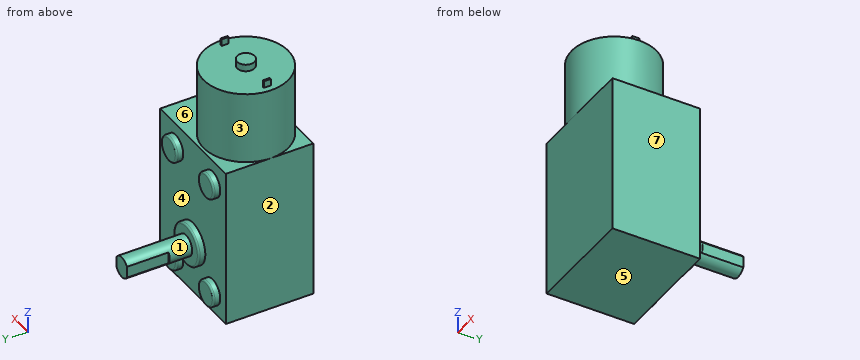
from build123d import *

# Parameters (mm, degrees)
CROQUIS1_W              = 32
CROQUIS1_H              = 46
CROQUIS1_R              = 6
CROQUIS1_R_2            = 3.7
SALIENTE_EXTRUIR1_DEPTH = 25.2
CROQUIS2_R              = 3.7
CROQUIS2_R_2            = 6
SALIENTE_EXTRUIR2_DEPTH = 2
CROQUIS3_R              = 12.2
SALIENTE_EXTRUIR3_DEPTH = 20.8
CROQUIS4_R              = 2.5
SALIENTE_EXTRUIR4_DEPTH = 2
CROQUIS5_W              = 0.5
CROQUIS5_H              = 2
SALIENTE_EXTRUIR5_DEPTH = 2
CROQUIS6_R              = 3
SALIENTE_EXTRUIR6_DEPTH = 18.5
CORTAR_EXTRUIR1_DEPTH   = 12
REDONDEO2_R             = 0.5


with BuildPart() as part:
    # Croquis1 → Saliente-Extruir1 (new body)
    with BuildSketch(Plane(origin=(0, 0, 0), x_dir=(1, 0, 0), z_dir=(0, 1, 0))):
        Rectangle(CROQUIS1_W, CROQUIS1_H)
        with Locations((0, 8)):
            Circle(CROQUIS1_R, mode=Mode.SUBTRACT)
        with Locations((8.430868167, -16)):
            Circle(CROQUIS1_R_2, mode=Mode.SUBTRACT)
        with Locations((-9.569131833, -16)):
            Circle(CROQUIS1_R_2, mode=Mode.SUBTRACT)
        with Locations((8.430868167, 17)):
            Circle(CROQUIS1_R_2, mode=Mode.SUBTRACT)
        with Locations((-9.569131833, 17)):
            Circle(CROQUIS1_R_2, mode=Mode.SUBTRACT)
        with Locations((0, 8)):
            Circle(CROQUIS1_R)
        with Locations((-9.569131833, 17)):
            Circle(CROQUIS1_R_2)
        with Locations((8.430868167, 17)):
            Circle(CROQUIS1_R_2)
        with Locations((-9.569131833, -16)):
            Circle(CROQUIS1_R_2)
        with Locations((8.430868167, -16)):
            Circle(CROQUIS1_R_2)
    extrude(amount=SALIENTE_EXTRUIR1_DEPTH)

    # Croquis2 → Saliente-Extruir2 (add)
    with BuildSketch(Plane(origin=(0, 25.2, 0), x_dir=(1, 0, 0), z_dir=(0, 1, 0))):
        with Locations((-9.569131833, 17)):
            Circle(CROQUIS2_R)
        with Locations((8.430868167, 17)):
            Circle(CROQUIS2_R)
        with Locations((8.430868167, -16)):
            Circle(CROQUIS2_R)
        with Locations((-9.569131833, -16)):
            Circle(CROQUIS2_R)
        with Locations((0, 8)):
            Circle(CROQUIS2_R_2)
    extrude(amount=SALIENTE_EXTRUIR2_DEPTH)

    # Croquis3 → Saliente-Extruir3 (add)
    with BuildSketch(Plane.XY.offset(23)):
        with Locations((-3.8, 12.2)):
            Circle(CROQUIS3_R)
    extrude(amount=SALIENTE_EXTRUIR3_DEPTH)

    # Croquis4 → Saliente-Extruir4 (add)
    with BuildSketch(Plane.XY.offset(43.8)):
        with Locations((-3.8, 12.2)):
            Circle(CROQUIS4_R)
    extrude(amount=SALIENTE_EXTRUIR4_DEPTH)

    # Croquis5 → Saliente-Extruir5 (add)
    with BuildSketch(Plane.XY.offset(43.8)):
        with Locations((6.559315441, 12.2)):
            Rectangle(CROQUIS5_W, CROQUIS5_H)
        with Locations((-13.968008184, 12.2)):
            Rectangle(CROQUIS5_W, CROQUIS5_H)
    extrude(amount=SALIENTE_EXTRUIR5_DEPTH)

    # Croquis6 → Saliente-Extruir6 (add)
    with BuildSketch(Plane(origin=(0, 27.2, 0), x_dir=(1, 0, 0), z_dir=(0, 1, 0))):
        with Locations((0, 8)):
            Circle(CROQUIS6_R)
    extrude(amount=SALIENTE_EXTRUIR6_DEPTH)

    # Croquis7 → Cortar-Extruir1 (cut)
    with BuildSketch(Plane(origin=(0, 45.7, 0), x_dir=(1, 0, 0), z_dir=(0, 1, 0))):
        with BuildLine():
            Line((-2.5, 6.341687605), (-2.5, 9.658312395))
            ThreePointArc((-2.5, 9.658312395), (-3, 8), (-2.5, 6.341687605))
        make_face()
        with BuildLine():
            Line((2.5, 6.341687605), (2.5, 9.658312395))
            ThreePointArc((2.5, 9.658312395), (3, 8), (2.5, 6.341687605))
        make_face()
    extrude(amount=-CORTAR_EXTRUIR1_DEPTH, mode=Mode.SUBTRACT)

    # Redondeo2
    redondeo2_edges = [part.edges().sort_by_distance(p)[0] for p in [
        (-13.269131833, 27.2, -17),
        (4.730868167, 27.2, -17),
        (4.730868167, 27.2, 16),
        (-13.269131833, 27.2, 16),
        (-6, 27.2, -8),
    ]]
    fillet(redondeo2_edges, radius=REDONDEO2_R)


solid = part.part
CAD build for the part. Positions are in the model's coordinates, mm. Face numbers are marked on the shaded views. A direction names the side the tool comes from. Give positions to 0.01 mm unless a question says otherwise; leave off trailing zeros. Write each loop counter-clockwise with the first axis right and the second up, starting at its lowest first coordinate (ties: lowest second). Pieces come first, ordered by that corner, then holes. Notation, with made-up numbers: (-38.75, 43) - (-17.75, 43) arc R16 ccw to (-17.75, 52) - close; hole circle Ø4 at (42, 4). An arc over 180 degrees is marked (long way). Put each result on its own line as item: value.
(1) Drop flat-ended pins along their axis: pin 1 Ø10 at (x, y) = (-7, 21.5) entering from +Z; pin 2 Ø7 at (x, z) = (-10.5, -16.5) entering from +Y; pin 3 Ø1.6 at (y, z) = (12.5, 45) entering from +X. Give the stop position or say it passes through.
Working result:
pin 1: z = 43.8
pin 2: y = 27.2
pin 3: x = 6.81
(2) Saw through at A-A (z = 16). List the corners of the cut face in (x, y), then the cut area to 3 significant figures.
Working result:
outline: (-16, 0) - (16, 0) - (16, 25.2) - (12.13, 25.2) - (12.13, 26.7) arc R0.5 ccw to (11.63, 27.2) - (5.23, 27.2) arc R0.5 ccw to (4.73, 26.7) - (4.73, 25.2) - (-5.87, 25.2) - (-5.87, 26.7) arc R0.5 ccw to (-6.37, 27.2) - (-12.77, 27.2) arc R0.5 ccw to (-13.27, 26.7) - (-13.27, 25.2) - (-16, 25.2) - close
area: 836 mm^2
(3) Tool access for the marked faces 1, 2 and 3: list every direction of +Z, -Z, +X, -X, +Y, -Y with a clear straight run to the whole face (end or side of a thin tool).
Working result:
face 1: +Y
face 2: +Z, -Z, -X, +Y, -Y
face 3: +Z
(4) Saw through at C-C (x = 0). List the corners of the cut face in (y, z).
Working result:
outline: (0, -23) - (25.2, -23) - (25.2, -14) - (26.7, -14) arc R0.5 ccw to (27.2, -13.5) - (27.2, -11) - (45.7, -11) - (45.7, -5) - (27.2, -5) - (27.2, -2.5) arc R0.5 ccw to (26.7, -2) - (25.2, -2) - (25.2, 23) - (23.79, 23) - (23.79, 43.8) - (0.61, 43.8) - (0.61, 23) - (0, 23) - close
(5) Wall check: L1, parallel to Z at x = -4, y = 16.5; L2, parallel to Z at x = 10, y = 24.5; L3, parallel to Y at x = 8, z = -15. Give the ranges that are in metal, low to high.
Working result:
L1: -23 to 43.8
L2: -23 to 23
L3: 0 to 27.2
(6) Saw through at D-D (z = -8). List the corners of the cut face in (x, y), then the cut area to 3 significant figures.
Working result:
outline: (-16, 0) - (16, 0) - (16, 25.2) - (6, 25.2) - (6, 26.7) arc R0.5 ccw to (5.5, 27.2) - (3, 27.2) - (3, 33.7) - (2.5, 33.7) - (2.5, 45.7) - (-2.5, 45.7) - (-2.5, 33.7) - (-3, 33.7) - (-3, 27.2) - (-5.5, 27.2) arc R0.5 ccw to (-6, 26.7) - (-6, 25.2) - (-16, 25.2) - close
area: 929 mm^2
(7) Pull direction Z, two halves, no side cores. Call the marked faces 4, 5, 6 and 7: released by +Z, released by -Z, zero draft, split by the parting line, or undercut.
Working result:
face 4: undercut
face 5: released by -Z
face 6: released by +Z
face 7: zero draft
(8) Saw through at B-B (y = 4). List the corners of the cut face in (x, z).
Working result:
outline: (-16, -23) - (16, -23) - (16, 23) - (5.23, 23) - (5.23, 43.8) - (-12.83, 43.8) - (-12.83, 23) - (-16, 23) - close
